```python
from build123d import *

# Parameters (mm, degrees)
F0_W      = 279.4
F0_H      = 101.6
F1_DEPTH  = 3.175
F2_W      = 25.4
F2_H      = 76.2
F3_DEPTH  = 3.176
F4_W      = 12.192
F4_H      = 21.082
F5_DEPTH  = 3.175
F7_D      = 6.6
F9_D      = 8.8
F11_D     = 8.8
F13_D     = 6.6
F14_W     = 25.4
F14_H     = 3.175
F15_DEPTH = 25.4
F17_D     = 6.6
F19_D     = 9
F20_D     = 6.6


with BuildPart() as f1:
    # F0 (on Top) → F1 (new body)
    with BuildSketch(Plane.XY):
        with Locations((37.6198536942, 37.7514991719)):
            Rectangle(F0_W, F0_H)
    extrude(amount=F1_DEPTH)

    # F2 (on face) → F3 (cut, through all)
    with BuildSketch(Plane.XY.offset(3.175)):
        with Locations((-89.3801463058, 25.0514991719)):
            Rectangle(F2_W, F2_H)
    extrude(amount=-F3_DEPTH, mode=Mode.SUBTRACT)

    # F4 (on face) → F5 (join)
    with BuildSketch(Plane(origin=(0, 0, 0), x_dir=(1, 0, 0), z_dir=(0, 0, -1))):
        with Locations((-45.1841463058, 23.5895008281)):
            Rectangle(F4_W, F4_H)
        Polygon((-39.0881463058, 13.0485008281), (-51.2801463058, 13.0485008281), (-76.6801463058, 13.0485008281), (-76.6801463058, -63.1514991719), (-102.0801463058, -63.1514991719), (-102.0801463058, -88.5514991719), (177.3198536942, -88.5514991719), (177.3198536942, 13.0485008281), align=None)
    extrude(amount=-F5_DEPTH)

    # F7 (through all)
    with Locations(Plane.XY.offset(3.175)):
        with Locations((-89.3801463058, 75.8514991719)):
            Hole(F7_D / 2)

    # F9 (through all)
    with Locations(Plane.XY.offset(3.175)):
        with Locations((-63.9801463058, 75.8514991719)):
            Hole(F9_D / 2)

    # F11 (through all)
    with Locations(Plane.XY.offset(3.175)):
        with Locations((-63.9801463058, -0.3485008281), (164.6198536942, -0.3485008281), (164.6198536942, 75.8514991719)):
            Hole(F11_D / 2)

    # F13 (through all)
    with Locations(Plane.XY.offset(3.175)):
        with Locations((-45.1841463058, -24.7325008281)):
            Hole(F13_D / 2)

    # F14 (on face) → F15 (join)
    with BuildSketch(Plane.YZ.offset(177.3198536942)):
        with Locations((75.8514991719, 1.5875)):
            Rectangle(F14_W, F14_H)
    extrude(amount=F15_DEPTH)

    # F17 (through all)
    with Locations(Plane(origin=(0, 0, 0), x_dir=(1, 0, 0), z_dir=(0, 0, -1))):
        with Locations((190.0198536942, -75.8514991719)):
            Hole(F17_D / 2)

    # F19 (through all)
    with Locations(Plane.XY.offset(3.175)):
        with Locations((-32.2301463058, 72.6764991719), (9.0448536942, 72.6764991719), (50.3198536942, 72.6764991719), (91.5948536942, 72.6764991719), (132.8698536942, 72.6764991719), (132.8698536942, 2.8264991719), (91.5948536942, 2.8264991719), (50.3198536942, 2.8264991719), (9.0448536942, 2.8264991719), (-32.2301463058, 2.8264991719)):
            Hole(F19_D / 2)

    # F20 (through all)
    with Locations(Plane.XY.offset(3.175)):
        with Locations((-32.2301463058, 59.8764993719), (9.0448536942, 59.8764993719), (50.3198536942, 59.8764993719), (91.5948536942, 59.8764993719), (132.8698536942, 59.8764993719), (132.8698536942, 15.6264989719), (91.5948536942, 15.6264989719), (50.3198536942, 15.6264989719), (9.0448536942, 15.6264989719), (-32.2301463058, 15.6264989719)):
            Hole(F20_D / 2)


solid = f1.part
```
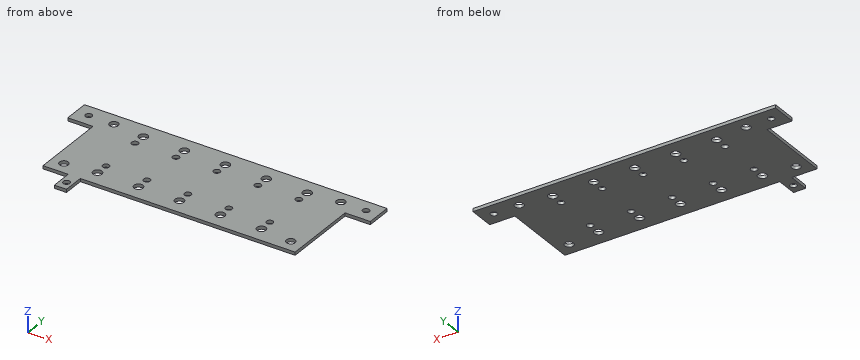
Check sheet for the modelled part. Datum: model origin and axes. Units: mm. Give positions to 0.01 mm unless a question says otherwise; leave off trailing zeros. Order: outer loops, then holes, each group sorted by start corner. A loop starts at its lowest first (then second) coordinate and runs counter-clockwise, first axis right, second up. Notation, with made-up numbers: M 58.25,16.25 L 80.25,16.25 A13 cw 80.25,30.25 Z; hole C 72,62.5 d6. An arc over 180 degrees is marked long. Answer in a Markdown table with one row per item.
1) Cross-section at B-B, the plane y = -16. Enter the section's corners in (x, z) (3 decimals).
Filled sheet:
| item | result |
|---|---|
| outline | M -51.28,0 L -39.088,0 L -39.088,3.175 L -51.28,3.175 Z |
2) Cross-section at D-D, the plane z = 0.95. Count the separate pieces of the cut face and the enclosed holes in it, plus the area to 3 significant figures.
Filled sheet:
| item | result |
|---|---|
| separate pieces | 1 |
| enclosed holes | 27 |
| area | 26,000 mm2 |
3) Cross-section at A-A, the plane x = -63.5. Enter the section's corners in (y, z) (1 decimal).
Filled sheet:
| item | result |
|---|---|
| outline | M -13,0 L -4.7,0 L -4.7,3.2 L -13,3.2 Z; M 4,0 L 71.5,0 L 71.5,3.2 L 4,3.2 Z; M 80.2,0 L 88.6,0 L 88.6,3.2 L 80.2,3.2 Z |
4) Gauge pin test, flat ends, axial feed: P1, Ø11.5, axis at x = 132.87, y = 72.68, coming from the +Z side (3 decimals); P2, Ø1, axis at x = -84.5, z = 2, coming from the -Y side. Record the tip position at first contact, or that the pin passes through.
Filled sheet:
| item | result |
|---|---|
| P1 | stops at z = 3.175 |
| P2 | stops at y = 63.15 |
5) Cross-section at C-C, the plane x = 62. Enter the section's corners in (y, z) (1 decimal), plus the area to 3 significant figures.
Filled sheet:
| item | result |
|---|---|
| outline | M -13,0 L 88.6,0 L 88.6,3.2 L -13,3.2 Z |
| area | 323 mm2 |
6) Thickness scan on L1, parallel to X at y = 16, z = 1.75; L2, parallel to X at y = 18, z = 1.6; L3, parallel to Y at x = 20, z = 2.2. Record the ranges inside material, lowest first. Write a range as [from, to].
Filled sheet:
| item | result |
|---|---|
| L1 | x = [-76.68, -35.51], [-28.95, 5.77], [12.32, 47.04], [53.6, 88.32], [94.87, 129.59], [136.15, 177.32] |
| L2 | x = [-76.68, -34.52], [-29.94, 6.75], [11.34, 48.03], [52.61, 89.3], [93.89, 130.58], [135.16, 177.32] |
| L3 | y = [-13.05, 88.55] |
